```python
from build123d import *
from build123d.topology import SkipClean

# Parameters (mm, degrees)
EXTRUDE_1_DEPTH     = 1.5
SKETCH_2_R          = 3.5
EXTRUDE_2_DEPTH     = 2.3
SKETCH_3_R          = 2.25
CUT_EXTRUDE_1_DEPTH = 3.8
SKETCH_5_R          = 0.5
CUT_EXTRUDE_2_DEPTH = 1.5


with BuildPart() as part:
    # 草图1 → 凸台-拉伸1 (new body)
    with BuildSketch(Plane.XY):
        with BuildLine():
            Line((-14.706896552, 1.485662753), (-0.482758621, 3.466546425))
            ThreePointArc((-0.482758621, 3.466546425), (0, 3.5), (0.482758621, 3.466546425))
            Line((0.482758621, 3.466546425), (14.706896552, 1.485662753))
            ThreePointArc((14.706896552, 1.485662753), (16, 0), (14.706896552, -1.485662753))
            Line((14.706896552, -1.485662753), (0.482758621, -3.466546425))
            ThreePointArc((0.482758621, -3.466546425), (0, -3.5), (-0.482758621, -3.466546425))
            Line((-0.482758621, -3.466546425), (-14.706896552, -1.485662753))
            ThreePointArc((-14.706896552, -1.485662753), (-16, 0), (-14.706896552, 1.485662753))
        make_face()
    extrude(amount=EXTRUDE_1_DEPTH)

    # 草图2 → 凸台-拉伸2 (add)
    with SkipClean():  # the faces are left unmerged after this step: merging them gives an invalid solid
        with BuildSketch(Plane.XY.offset(1.5)):
            with Locations(Location((0, 0, 0), (0, 0, 97.928141766))):
                Circle(SKETCH_2_R)
        extrude(amount=EXTRUDE_2_DEPTH)
    add(part.part.scale(1), mode=Mode.REPLACE)  # the faces are merged on a copy

    # 草图3 → 切除-拉伸1 (cut)
    with BuildSketch(Plane.XY.offset(3.8)):
        Circle(SKETCH_3_R)
    extrude(amount=-CUT_EXTRUDE_1_DEPTH, mode=Mode.SUBTRACT)

    # 草图5 → 切除-拉伸2 (cut)
    with BuildSketch(Plane(origin=(0, 0, 0), x_dir=(-1, 0, 0), z_dir=(0, 0, -1))):
        with Locations((-4.5, 0)):
            Circle(SKETCH_5_R)
        with Locations((-6.5, 0)):
            Circle(SKETCH_5_R)
        with Locations((-8.5, 0)):
            Circle(SKETCH_5_R)
        with Locations((-10.5, 0)):
            Circle(SKETCH_5_R)
        with Locations((-12.5, 0)):
            Circle(SKETCH_5_R)
        with Locations((-14.5, 0)):
            Circle(SKETCH_5_R)
        with Locations(Location((4.5, 0, 0), (0, 0, 180))):
            Circle(SKETCH_5_R)
        with Locations(Location((14.5, 0, 0), (0, 0, 180))):
            Circle(SKETCH_5_R)
        with Locations(Location((12.5, 0, 0), (0, 0, 180))):
            Circle(SKETCH_5_R)
        with Locations(Location((10.5, 0, 0), (0, 0, 180))):
            Circle(SKETCH_5_R)
        with Locations(Location((8.5, 0, 0), (0, 0, 180))):
            Circle(SKETCH_5_R)
        with Locations(Location((6.5, 0, 0), (0, 0, 180))):
            Circle(SKETCH_5_R)
    extrude(amount=-CUT_EXTRUDE_2_DEPTH, mode=Mode.SUBTRACT)


solid = part.part
```
Read the model definition and answer for the solid it produces. Units are mm, in the model's axes. Round coordinates to 2 decimals unless told otherwise and drop trailing zeros. Write each loop counter-clockwise with the first axis right and the second up, starting at its lowest first coordinate (ties: lowest second). Pieces come first, ordered by that corner, then holes. Notation, with made-up numbers: (-22, 63) - (0, 63) arc R18 cw to (0, 73) - close; hole circle Ø4 at (53, 70.25). An arc over 180 degrees is marked (long way). One line per item, written item: value.
Q1. Find section A-A (z = 0.7). Count the separate pieces of the cut face and the enclosed holes in it, and give its area (3 significant figures).
The answers:
separate pieces: 1
enclosed holes: 13
area: 128 mm2
Q2. Find section B-B (x = 0). Determine the outline of the cut face in (y, z).
The answers:
outline: (-3.5, 0) - (-2.25, 0) - (-2.25, 3.8) - (-3.5, 3.8) - close; (2.25, 0) - (3.5, 0) - (3.5, 3.8) - (2.25, 3.8) - close
Q3. Each of these flat-tipped pins is pushed along its axis until it touches: P1, Ø1.5, axis at y = 1, z = 3, coming from the +X side; P2, Ø2, axis at x = 8.5, z = 3.5, coming from the +Y side; P3, Ø2, axis at y = -0.5, z = 3, coming from the -X side; P4, Ø3.5, axis at x = -9.5, y = 1, coming from the +Z side. Where does it stop, or does it pass through?
The answers:
P1: stops at x = 3.49
P2: passes through
P3: stops at x = -3.5
P4: stops at z = 1.5
Q4. Find section C-C (z = 2.05). Determine the outline of the cut face in (x, y), and give its area (3 significant figures).
The answers:
outline: circle Ø7 at (0, 0); hole circle Ø4.5 at (0, 0)
area: 22.6 mm2
Q5. Straight lines are drawn through the part: line 1 (Z direction, x = 10, y = 0.5); line 2 (X direction, y = 0.5, z = 2.45); line 3 (Y direction, x = -14.5, z = 1.1). For each, find the intervals that lie inside material, in ascending order. Write a range as from..to.
The answers:
line 1: z = 0..1.5
line 2: x = -3.46..-2.19, 2.19..3.46
line 3: y = -1.51..-0.5, 0.5..1.51
Q6. For a pull along Y with two mould halves and no side action, classify faces 1 (the cylindrical face through (8, 0, 1)), 2 (the cylindrical face through (-5, 0, 1)), 3 (the cylindrical face through (16, 0, 1)), 4 (the flat face through (8, -1, 1.5)) as pulls with the +Y half, pulls with the -Y half, needs draft (parallel to the pull), parting line crosses it, or undercut.
The answers:
face 1: undercut
face 2: undercut
face 3: parting line crosses it
face 4: needs draft
Q7. Find section D-D (x = 6.5). Determine the outline of the cut face in (y, z), and give its area (3 significant figures).
The answers:
outline: (-2.63, 0) - (-0.5, 0) - (-0.5, 1.5) - (-2.63, 1.5) - close; (0.5, 0) - (2.63, 0) - (2.63, 1.5) - (0.5, 1.5) - close
area: 6.39 mm2
